Verification items for the finished model (mm, model axes). A direction names the side the tool comes from. Round coordinates to 2 decimals unless told otherwise and drop trailing zeros. Write each loop counter-clockwise with the first axis right and the second up, starting at its lowest first coordinate (ties: lowest second). Pieces come first, ordered by that corner, then holes.
from build123d import *

# Parameters (mm, degrees)
F1_DEPTH = 10
F2_DEPTH = 12
F4_DEPTH = 25


with BuildPart() as f1:
    # F0 (on Top) → F1 (new body)
    with BuildSketch(Plane.XY):
        Polygon((2, -5.5), (2, 0), (10.000001, 0), (12.000001, 0), (12.000001, 2), (10.000001, 2), (0, 2), (0, 0), (0, -5.5), align=None)
        Polygon((2, -5.7), (2, -5.5), (0, -5.5), (0, -5.7), (0, -7.7), (10.000001, -7.7), (12.000001, -7.7), (12.000001, -5.7), (10.000001, -5.7), align=None)
    extrude(amount=F1_DEPTH)

    # F0 (on Top) → F2 (join)
    with BuildSketch(Plane.XY):
        Polygon((0, -5.7), (0, -5.5), (-7.940744, -5.5), (-13.940744, -5.5), (-16, -5.5), (-17, -5.5), (-17, -7.7), (-16, -7.7), (-15, -7.7), (-10, -7.7), (-7.940744, -7.7), (0, -7.7), align=None)
    extrude(amount=F2_DEPTH)

    # F3 (on face) → F4 (cut)
    with BuildSketch(Plane(origin=(0, -5.5, 0), x_dir=(-1, 0, 0), z_dir=(0, 1, 0))):
        with BuildLine():
            ThreePointArc((1.89697, 12), (7.060791, 2.145721), (15.68, 9.18))
            ThreePointArc((15.68, 9.18), (15.534279, 10.619209), (15.10303, 12))
            Line((15.10303, 12), (1.89697, 12))
        make_face()
    extrude(amount=-F4_DEPTH, mode=Mode.SUBTRACT)


solid = f1.part
Q1. Sectioned sample at C-C (z = 1). Enter the section's corners in (x, y), plus the area to 3 significant figures.
Recorded:
outline: (-17, -7.7) - (12, -7.7) - (12, -5.7) - (2, -5.7) - (2, 0) - (12, 0) - (12, 2) - (0, 2) - (0, -5.5) - (-17, -5.5) - close
area: 96.8 mm2
Q2. Depth check by flat-ended pin: P1, Ø1.5, axis at x = 6.5, y = -3, coming from the -Z side; P2, Ø3, axis at x = 8.5, y = -4.5, coming from the +Z side; P3, Ø1.7, axis at y = -2.5, z = 7.5, coming from the +X side; P4, Ø1, axis at x = -5, z = 3, coming from the -Y side. Enter the tip coordinate at first touch or a pass-through.
Recorded:
P1: passes through
P2: stops at z = 10
P3: stops at x = 2
P4: stops at y = -7.7
Q3. Release check for a two-part mould opening along Y. For faces 5 (the flat face through (1, -7.7, 5)), 6 (the flat face through (2, -3, 5)), 7 (the flat face through (4.6, 0.5, 10)) record: released by +Y, released by -Y, zero draft, split by the parting line, or undercut.
Recorded:
face 5: released by -Y
face 6: undercut
face 7: zero draft
Q4. Tool access check on faces 1 (the flat face through (0, -7, 11)), 2 (the flat face through (-6, -5.5, 2)), 3 (the flat face through (6, 2, 5)), 4 (the flat face through (7, -5.7, 5)). Record the directions out of +Z, -Z, +X, -X, +Y, -Y that give a thin tool (end or side, any length) a straight path to the whole face; none if there is none.
Recorded:
face 1: +Z, +X, +Y, -Y
face 2: +Z, -Z, -X, +Y
face 3: +Z, -Z, +X, -X, +Y
face 4: +Z, -Z, +X
Q5. Sectioned sample at B-B (z = 4.5). Enter the section's corners in (x, y), plus the area to 3 significant figures.
Recorded:
outline: (-17, -7.7) - (-13.95, -7.7) - (-13.95, -5.5) - (-17, -5.5) - close; (-3.05, -7.7) - (12, -7.7) - (12, -5.7) - (2, -5.7) - (2, 0) - (12, 0) - (12, 2) - (0, 2) - (0, -5.5) - (-3.05, -5.5) - close
area: 72.8 mm2
Q6. Sectioned sample at A-A (x = 2.75). Enter the section's corners in (y, z), plus the area to 3 significant figures.
Recorded:
outline: (-7.7, 0) - (-5.7, 0) - (-5.7, 10) - (-7.7, 10) - close; (0, 0) - (2, 0) - (2, 10) - (0, 10) - close
area: 40.0 mm2
Q7. Sectioned sample at D-D (z = 6.25). Enter the section's corners in (x, y), plus the area to 3 significant figures.
Recorded:
outline: (-17, -7.7) - (-15.05, -7.7) - (-15.05, -5.5) - (-17, -5.5) - close; (-1.95, -7.7) - (12, -7.7) - (12, -5.7) - (2, -5.7) - (2, 0) - (12, 0) - (12, 2) - (0, 2) - (0, -5.5) - (-1.95, -5.5) - close
area: 68.0 mm2
Q8. Material ranges on line 1 along Y through (x, z) = (3.25, 4.5); line 2 along X through (y, z) = (-6.7, 9.18); line 3 along Y through (x, z) = (-3.25, 0.75), recorded low to high.
Recorded:
line 1: y = -7.7 to -5.7, 0 to 2
line 2: x = -17 to -15.68, -1.32 to 12
line 3: y = -7.7 to -5.5
